from build123d import *

# Parameters (mm, degrees)
SKETCH1_W           = 12
SKETCH1_H           = 13
BOSS_EXTRUDE1_DEPTH = 5
SKETCH3_R           = 6.5
CUT_EXTRUDE1_DEPTH  = 9
SKETCH4_R           = 1.75
CUT_EXTRUDE2_DEPTH  = 3
FILLET1_START       = -1
FILLET1_DEPTH       = 7
FILLET2_R           = 1.5


with BuildPart() as part:
    # Sketch1 → Boss-Extrude1 (new body)
    with BuildSketch(Plane.XY):
        with Locations((6, 6.5)):
            Rectangle(SKETCH1_W, SKETCH1_H)
    extrude(amount=BOSS_EXTRUDE1_DEPTH)

    # Sketch3 → Cut-Extrude1 (cut)
    with BuildSketch(Plane.XY.offset(5)):
        with Locations((12, 6.5)):
            Circle(SKETCH3_R)
    extrude(amount=-CUT_EXTRUDE1_DEPTH, mode=Mode.SUBTRACT)

    # Sketch4 → Cut-Extrude2 (cut)
    with BuildSketch(Plane.ZY):
        with Locations((2.5, 6.5)):
            Circle(SKETCH4_R)
    extrude(amount=-CUT_EXTRUDE2_DEPTH, mode=Mode.SUBTRACT)

    # Fillet1: read off the stored shape, not the designer's step
    # Fillet1 outline → Fillet1 (cut)
    with BuildSketch(Plane.XY.offset(FILLET1_START)):
        with BuildLine():
            ThreePointArc((5.755002002, 13), (7.10708373, 12.149519053), (6.925939126, 10.5625))
            ThreePointArc((6.925939126, 10.5625), (9.185417438, 12.359020823), (12, 13))
            Line((12, 13), (5.755002002, 13))
        make_face()
        with BuildLine():
            ThreePointArc((6.925939126, 2.4375), (7.10708373, 0.850480947), (5.755002002, 0))
            Line((5.755002002, 0), (12, 0))
            ThreePointArc((12, 0), (9.185417438, 0.640979177), (6.925939126, 2.4375))
        make_face()
    extrude(amount=FILLET1_DEPTH, mode=Mode.SUBTRACT)

    # Fillet2
    fillet2_edges = [part.edges().sort_by_distance(p)[0] for p in [
        (0, 13, 2.5),
        (0, 0, 2.5),
    ]]
    fillet(fillet2_edges, radius=FILLET2_R)


solid = part.part
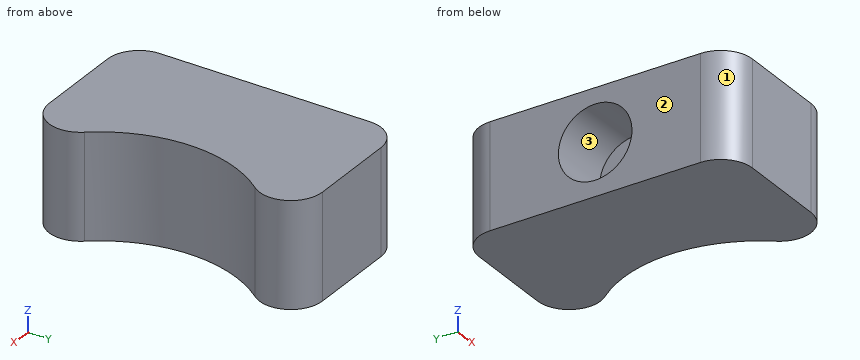
Could you check a few things on this model? Use its own coordinates, in mm. Face numbers are marked on the shaded views. Round coordinates to 2 decimals unless told otherwise and drop trailing zeros. Write each loop counter-clockwise with the first axis right and the second up, starting at its lowest first coordinate (ties: lowest second). Pieces come first, ordered by that corner, then holes. Notation, with made-up numbers: (14, 38.25) -> (22, 38.25) arc R17 cw to (22, 59.25) -> close; hole circle Ø3 at (34.5, 31.25). An arc over 180 degrees is marked (long way). Use a Markdown table: item, result.
1. If we section it at A-A (x = 6.25): List the corners of the cut face in (y, z) for me, then the cut area to 3 significant figures.
Answer key:
| item | result |
|---|---|
| outline | (0.08, 0) -> (3.47, 0) -> (3.47, 5) -> (0.08, 5) -> close; (9.53, 0) -> (12.92, 0) -> (12.92, 5) -> (9.53, 5) -> close |
| area | 33.8 mm^2 |
2. If we section it at D-D (x = 2.5): List the corners of the cut face in (y, z) for me.
Answer key:
| item | result |
|---|---|
| outline | (0, 0) -> (13, 0) -> (13, 5) -> (0, 5) -> close; hole circle Ø3.5 at (6.5, 2.5) |
3. Please list where these lines run through material, in increasing order: probe 1 along Y at (x, z) = (2.4, 2.5); probe 2 along Z at (x, y) = (2.5, 7.5); probe 3 along X at (y, z) = (8.75, 1.25).
Answer key:
| item | result |
|---|---|
| probe 1 | y = 0 to 4.75, 8.25 to 13 |
| probe 2 | z = 0 to 1.06, 3.94 to 5 |
| probe 3 | x = 0 to 5.9 |
4. For pin 1 Ø2 at (y, z) = (7, 1) entering from +X, with a flat end and sliding along its axis, tell me the tip position at first contact or that it passes through.
Answer key:
| item | result |
|---|---|
| pin 1 | stops at x = 5.68 |
5. If we section it at B-B (y = 6.5): List the corners of the cut face in (x, z) for me, then the cut area to 3 significant figures.
Answer key:
| item | result |
|---|---|
| outline | (0, 0) -> (5.5, 0) -> (5.5, 5) -> (0, 5) -> (0, 4.25) -> (3, 4.25) -> (3, 0.75) -> (0, 0.75) -> close |
| area | 17.0 mm^2 |
6. We'd pull the mould along Y, two halves only. Please class the marked faces 1, 2 and 3: +Y half, -Y half, draft (parallel to the pull), parting line (faces both ways), or undercut.
Answer key:
| item | result |
|---|---|
| face 1 | -Y half |
| face 2 | draft |
| face 3 | undercut |
